Read the model definition and answer for the solid it produces. Units are mm, in the model's axes. A direction names the side the tool comes from. Coordinates: 2 decimals unless noted, no trailing zeros. Write each loop counter-clockwise with the first axis right and the second up, starting at its lowest first coordinate (ties: lowest second). Pieces come first, ordered by that corner, then holes.
(1) Find the intervals of material crossed by probe 1 along Y at (x, z) = (-9.5, -31); probe 2 along Z at (x, y) = (4.25, 50.5); probe 3 along Z at (x, y) = (2, 69.5), in increasing order.
(2) Section D-D on z = -15 is taken. Write down the section's boundary in (x, y), then the cut area to 3 significant figures.
(3) Section B-B on z = -8 is taken. Write down the section's boundary in (x, y).
(4) The mould has two halves that part along X. Classify faces 4 (the flat face through (13.263, 20, -36)), 5 (the cylindrical face through (-3.28, 46.97, -24.58)), 6 (the flat face through (-1, 4, 8.417)): +X half, -X half, draft (parallel to the pull), parting line (faces both ways), or undercut.
(5) Given pin 1 (5.5 mm diameter, centred on x = 8.65, z = -8.23, fed in from +Y); pin 2 (2.5 mm diameter, centred on x = 2, y = 48.5, fed in from +Z); pin 3 (8 mm diameter, centred on x = -2.5, z = -11, fed in from +Y); pin 4 (10.5 mm diameter, centred on x = 0.5, z = -26.5, fed in from -Y), each flat-ended and moving along its own axis, determine where each tip first touches the part or whether it passes through.
(6) Which of the six approach directions +Z, -Z, +X, -X, +Y, -Y give full straight-line access (tool end or side, diameter ignored) to faces 1 (the flat face through (-1, 7.62, -13)), 2 (the flat face through (-1, 53.34, -32)), 3 (the flat face through (11, 5.08, -8))?
(7) Section C-C on y = 67 is taken. Write down the section's boundary in (x, z), then the cut area to 3 significant figures.
(8) Section A-A on y = 47.5 is taken. Write down the section's boundary in (x, z).
from build123d import *

# Parameters (mm, degrees)
SKETCH1_W           = 27.22
SKETCH1_H           = 50.8
BOSS_EXTRUDE1_DEPTH = 7.62
SKETCH2_R           = 2.05
CUT_EXTRUDE1_DEPTH  = 7.62
SKETCH3_R           = 3.3782
CUT_EXTRUDE2_DEPTH  = 2.54
SKETCH4_W           = 27.22
SKETCH4_H           = 7.62
BOSS_EXTRUDE2_DEPTH = 45.72
SKETCH10_W          = 27.22
SKETCH10_H          = 7.62
BOSS_EXTRUDE3_DEPTH = 12.7
CUT_EXTRUDE6_DEPTH  = 7.62
SKETCH13_R          = 4.826
CUT_EXTRUDE7_DEPTH  = 2.54
SKETCH12_W          = 27.22
SKETCH12_H          = 3.81
BOSS_EXTRUDE4_DEPTH = 20.32


with BuildPart() as part:
    # Sketch1 → Boss-Extrude1 (new body)
    with BuildSketch(Plane(origin=(0, 0, 0), x_dir=(1, 0, 0), z_dir=(0, 1, 0))):
        with Locations((-0.346834532, 16.982733813)):
            Rectangle(SKETCH1_W, SKETCH1_H)
    extrude(amount=BOSS_EXTRUDE1_DEPTH)

    # Sketch2 → Cut-Extrude1 (cut)
    with BuildSketch(Plane(origin=(0, 7.62, 0), x_dir=(1, 0, 0), z_dir=(0, 1, 0))):
        with Locations(Location((-9.346834532, 8.232733813, 0), (0, 0, 270))):
            Circle(SKETCH2_R)
    cut_extrude1 = extrude(amount=-CUT_EXTRUDE1_DEPTH, mode=Mode.SUBTRACT)

    # Sketch3 → Cut-Extrude2 (cut)
    with BuildSketch(Plane(origin=(0, 7.62, 0), x_dir=(1, 0, 0), z_dir=(0, 1, 0))):
        with Locations(Location((-9.346834532, 8.232733813, 0), (0, 0, 270))):
            Circle(SKETCH3_R)
    cut_extrude2 = extrude(amount=-CUT_EXTRUDE2_DEPTH, mode=Mode.SUBTRACT)

    # Mirror1: Cut-Extrude1, Cut-Extrude2 across plane
    add(cut_extrude1.mirror(Plane.ZY.offset(0.346834532)), mode=Mode.SUBTRACT)
    add(cut_extrude2.mirror(Plane.ZY.offset(0.346834532)), mode=Mode.SUBTRACT)

    # Sketch4 → Boss-Extrude2 (add)
    with BuildSketch(Plane(origin=(0, 7.62, 0), x_dir=(1, 0, 0), z_dir=(0, 1, 0))):
        with Locations((-0.346834532, 38.572733813)):
            Rectangle(SKETCH4_W, SKETCH4_H)
    extrude(amount=BOSS_EXTRUDE2_DEPTH)

    # Sketch10 → Boss-Extrude3 (add)
    with BuildSketch(Plane.XY.offset(-34.762733813)):
        with Locations((-0.346834532, 49.53)):
            Rectangle(SKETCH10_W, SKETCH10_H)
    extrude(amount=BOSS_EXTRUDE3_DEPTH)

    # Sketch11 → Cut-Extrude6 (cut)
    with BuildSketch(Plane.XZ.offset(-45.72)):
        with BuildLine():
            ThreePointArc((2.955165468, -28.412733813), (1.988032059, -26.077867221), (-0.346834532, -25.110733813))
            Line((-0.346834532, -25.110733813), (-0.346834532, -31.714733813))
            ThreePointArc((-0.346834532, -31.714733813), (1.988032059, -30.747600404), (2.955165468, -28.412733813))
        make_face()
        with BuildLine():
            Line((-0.346834532, -31.714733813), (-0.346834532, -25.110733813))
            ThreePointArc((-0.346834532, -25.110733813), (-3.648834532, -28.412733813), (-0.346834532, -31.714733813))
        make_face()
    extrude(amount=-CUT_EXTRUDE6_DEPTH, mode=Mode.SUBTRACT)

    # Sketch13 → Cut-Extrude7 (cut)
    with BuildSketch(Plane.XZ.offset(-45.72)):
        with Locations(Location((-0.346834532, -28.412733813, 0), (0, 0, 270))):
            Circle(SKETCH13_R)
    extrude(amount=-CUT_EXTRUDE7_DEPTH, mode=Mode.SUBTRACT)

    # Sketch12 → Boss-Extrude4 (add)
    with BuildSketch(Plane(origin=(0, 53.34, 0), x_dir=(1, 0, 0), z_dir=(0, 1, 0))):
        with Locations((-0.346834532, 40.477733813)):
            Rectangle(SKETCH12_W, SKETCH12_H)
    extrude(amount=BOSS_EXTRUDE4_DEPTH)


solid = part.part
Response:
1. probe 1: y = 0 to 7.62, 45.72 to 53.34
1. probe 2: z = -42.38 to -22.06
1. probe 3: z = -42.38 to -38.57
2. outline: (-13.96, 0) - (13.26, 0) - (13.26, 7.62) - (-13.96, 7.62) - close
2. area: 207 mm2
3. outline: (-13.96, 0) - (-11.38, 0) - (-11.38, 5.08) - (-12.72, 5.08) - (-12.72, 7.62) - (-13.96, 7.62) - close; (-7.31, 0) - (6.62, 0) - (6.62, 5.08) - (5.28, 5.08) - (5.28, 7.62) - (-5.98, 7.62) - (-5.98, 5.08) - (-7.31, 5.08) - close; (10.69, 0) - (13.26, 0) - (13.26, 7.62) - (12.02, 7.62) - (12.02, 5.08) - (10.69, 5.08) - close
4. face 4: +X half
4. face 5: undercut
4. face 6: draft
5. pin 1: stops at y = 5.08
5. pin 2: stops at z = -22.06
5. pin 3: stops at y = 7.62
5. pin 4: stops at y = 0
6. face 1: +Z, +X, -X
6. face 2: +Z, +X, -X, +Y
6. face 3: +Y
7. outline: (-13.96, -42.38) - (13.26, -42.38) - (13.26, -38.57) - (-13.96, -38.57) - close
7. area: 104 mm2
8. outline: (-13.96, -42.38) - (13.26, -42.38) - (13.26, -22.06) - (-13.96, -22.06) - close; hole circle Ø9.65 at (-0.35, -28.41)
